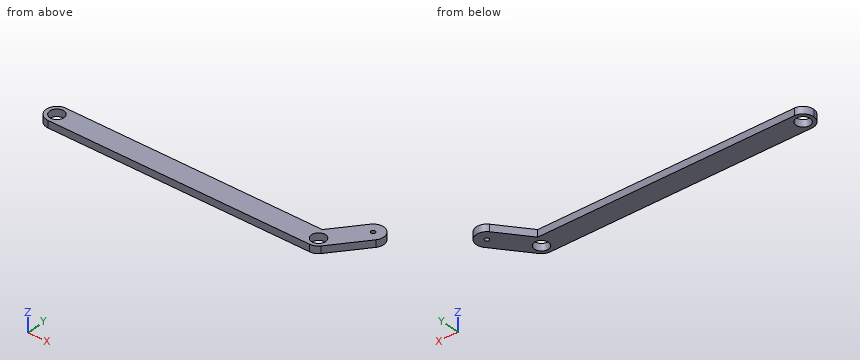
from build123d import *

# Parameters (mm, degrees)
SKETCH1_W           = 198
SKETCH1_H           = 15
BOSS_EXTRUDE1_DEPTH = 5
SKETCH2_R           = 5
CUT_EXTRUDE1_DEPTH  = 6
SKETCH3_R           = 1.5
BOSS_EXTRUDE2_DEPTH = 5


with BuildPart() as part:
    # Sketch1 → Boss-Extrude1 (new body)
    with BuildSketch(Plane.XY):
        with Locations((52.20591631, 1.643835616)):
            Rectangle(SKETCH1_W, SKETCH1_H)
    extrude(amount=BOSS_EXTRUDE1_DEPTH)

    # Sketch2 → Cut-Extrude1 (cut, through all)
    with BuildSketch(Plane.XY.offset(5)):
        with BuildLine():
            Line((-39.29408369, 9.143835616), (-46.79408369, 9.143835616))
            Line((-46.79408369, 9.143835616), (-46.79408369, 1.643835616))
            ThreePointArc((-46.79408369, 1.643835616), (-44.597384548, 6.947136475), (-39.29408369, 9.143835616))
        make_face()
        with BuildLine():
            ThreePointArc((-39.29408369, -5.856164384), (-44.597384548, -3.659465242), (-46.79408369, 1.643835616))
            Line((-46.79408369, 1.643835616), (-46.79408369, -5.856164384))
            Line((-46.79408369, -5.856164384), (-39.29408369, -5.856164384))
        make_face()
        with BuildLine():
            Line((151.20591631, 9.143835616), (143.70591631, 9.143835616))
            ThreePointArc((143.70591631, 9.143835616), (149.009217169, 6.947136475), (151.20591631, 1.643835616))
            Line((151.20591631, 1.643835616), (151.20591631, 9.143835616))
        make_face()
        with BuildLine():
            ThreePointArc((151.20591631, 1.643835616), (149.009217169, -3.659465242), (143.70591631, -5.856164384))
            Line((143.70591631, -5.856164384), (151.20591631, -5.856164384))
            Line((151.20591631, -5.856164384), (151.20591631, 1.643835616))
        make_face()
        with Locations((-39.29408369, 1.643835616)):
            Circle(SKETCH2_R)
        with Locations((143.70591631, 1.643835616)):
            Circle(SKETCH2_R)
    extrude(amount=-CUT_EXTRUDE1_DEPTH, mode=Mode.SUBTRACT)

    # Sketch3 → Boss-Extrude2 (add)
    with BuildSketch(Plane.XY.offset(5)):
        with BuildLine():
            ThreePointArc((143.70591631, 9.143835616), (150.486406082, 4.849293221), (149.50180231, -3.116175463))
            Line((149.50180231, -3.116175463), (168.541846628, 20.067368536))
            ThreePointArc((168.541846628, 20.067368536), (167.505971708, 30.623265615), (156.950074629, 29.587390695))
            Line((156.950074629, 29.587390695), (140.160312255, 9.143835616))
            Line((140.160312255, 9.143835616), (143.70591631, 9.143835616))
        make_face()
        with Locations((162.745960629, 24.827379616)):
            Circle(SKETCH3_R, mode=Mode.SUBTRACT)
    extrude(amount=-BOSS_EXTRUDE2_DEPTH)


solid = part.part
Part model, mm, in its own coordinate system. Round coordinates to 2 decimals unless told otherwise and drop trailing zeros. Write each loop counter-clockwise with the first axis right and the second up, starting at its lowest first coordinate (ties: lowest second). Pieces come first, ordered by that corner, then holes. Notation, with made-up numbers: M 29,66.5 L 68,66.5 A17 ccw 68,88.5 Z; hole C 84.5,46 d2. An arc over 180 degrees is marked long. Return JSON: item names as keys, results as strings. Group by question number.
(1) Pin check, flat tips, straight feed: pin 1 Ø1 at (x, z) = (-16.5, 3.5) entering from +Y; pin 2 Ø6 at (x, y) = (-39.29, 1.64) entering from -Z. Stop position of each tip, or through.
(2) Drill centre lines: probe 1 along X at (y, z) = (4.5, 0.45); probe 2 along Y at (x, z) = (13, 1.45); probe 3 along Y at (x, z) = (-36, 4.3). Where is each one in solid material? Low to high.
(3) Saw through at A-A on z = 3.15. Write the cut outline in (x, y).
(4) Saw through at C-C on y = 11. Write the cut outline in (x, z).
(5) Saw through at B-B on x = 46. Write the cut outline in (y, z).
Returned:
{
 "1": {"pin 1": "y = 9.14", "pin 2": "through"},
 "2": {"probe 1": "-46.23 to -43.4, -35.19 to 139.6, 147.81 to 155.76", "probe 2": "-5.86 to 9.14", "probe 3": "-5.86 to -2.12, 5.41 to 9.14"},
 "3": {"outline": "M -39.29,-5.86 L 143.71,-5.86 A7.5 ccw 149.5,-3.12 L 168.54,20.07 A7.5 ccw 156.95,29.59 L 140.16,9.14 L -39.29,9.14 A7.5 ccw Z; hole C -39.29,1.64 d10; hole C 143.71,1.64 d10; hole C 162.75,24.83 d3"},
 "4": {"outline": "M 141.68,0 L 161.1,0 L 161.1,5 L 141.68,5 Z"},
 "5": {"outline": "M -5.86,0 L 9.14,0 L 9.14,5 L -5.86,5 Z"}
}
